Here's how the part is built. I have some questions about the finished solid (model axes, mm). Face numbers are marked on the shaded views. Coordinates: 2 decimals unless noted, no trailing zeros. Write each loop counter-clockwise with the first axis right and the second up, starting at its lowest first coordinate (ties: lowest second). Pieces come first, ordered by that corner, then holes. Notation, with made-up numbers: M 15.25,-20 L 27.25,-20 A15 ccw 27.25,-2 Z; hole C 12.5,47.25 d6. An arc over 180 degrees is marked long. Use a Markdown table: item, result.
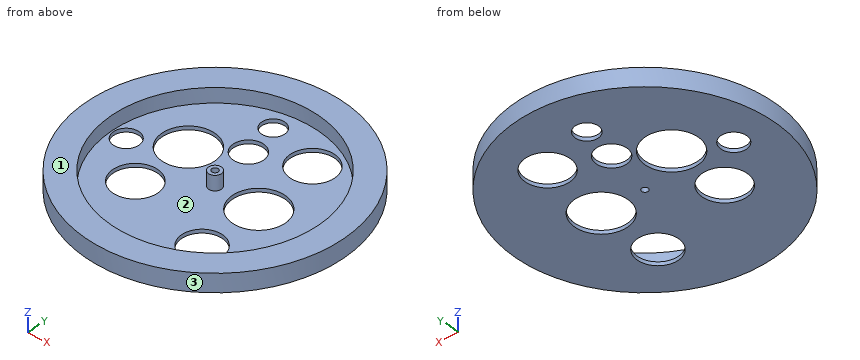
```python
from build123d import *

# Parameters (mm, degrees)
F0_R      = 70.662875
F1_DEPTH  = 10
F2_R      = 56.784897
F3_DEPTH  = 8
F4_R      = 14.477715
F5_DEPTH  = 8
F6_R      = 12.226907
F7_DEPTH  = 8
F8_R      = 7.014045
F9_DEPTH  = 8
F10_R     = 14.443937
F11_DEPTH = 8
F13_R     = 6.303091
F14_DEPTH = 8
F15_R     = 8.317638
F16_DEPTH = 8
F17_R     = 6.025281
F18_DEPTH = 8
F19_R     = 11.209177
F20_DEPTH = 8
F12_R     = 3.5
F21_DEPTH = 8
F23_D     = 3.5
F24_R     = 12.274082
F25_DEPTH = 8


with BuildPart() as f1:
    # F0 (on Top) → F1 (new body)
    with BuildSketch(Plane.XY):
        Circle(F0_R)
    extrude(amount=F1_DEPTH)

    # F2 (on face) → F3 (cut)
    with BuildSketch(Plane.XY.offset(10)):
        Circle(F2_R)
    extrude(amount=-F3_DEPTH, mode=Mode.SUBTRACT)

    # F4 (on face) → F5 (cut)
    with BuildSketch(Plane.XY.offset(2)):
        with Locations((-25.900649, 12.583426)):
            Circle(F4_R)
    extrude(amount=-F5_DEPTH, mode=Mode.SUBTRACT)

    # F6 (on face) → F7 (cut)
    with BuildSketch(Plane.XY.offset(2)):
        with Locations((20.854684, 36.710624)):
            Circle(F6_R)
    extrude(amount=-F7_DEPTH, mode=Mode.SUBTRACT)

    # F8 (on face) → F9 (cut)
    with BuildSketch(Plane.XY.offset(2)):
        with Locations((-48.892226, 0)):
            Circle(F8_R)
    extrude(amount=-F9_DEPTH, mode=Mode.SUBTRACT)

    # F10 (on face) → F11 (cut)
    with BuildSketch(Plane.XY.offset(2)):
        with Locations((24.09202, 0)):
            Circle(F10_R)
    extrude(amount=-F11_DEPTH, mode=Mode.SUBTRACT)

    # F13 (on face) → F14 (cut)
    with BuildSketch(Plane.XY.offset(2)):
        with Locations((-8.595636, 45.51062)):
            Circle(F13_R)
    extrude(amount=-F14_DEPTH, mode=Mode.SUBTRACT)

    # F15 (on face) → F16 (cut)
    with BuildSketch(Plane.XY.offset(2)):
        with Locations((-5.225664, 26.43148)):
            Circle(F15_R)
    extrude(amount=-F16_DEPTH, mode=Mode.SUBTRACT)

    # F17 (on Top) → F18 (cut)
    with BuildSketch(Plane.XY):
        with Locations((14.564808, -20.261167)):
            Circle(F17_R)
    extrude(amount=-F18_DEPTH, mode=Mode.SUBTRACT)

    # F19 (on face) → F20 (cut)
    with BuildSketch(Plane.XY.offset(2)):
        with Locations((23.249339, -34.03841)):
            Circle(F19_R)
    extrude(amount=-F20_DEPTH, mode=Mode.SUBTRACT)

    # F12 (on face) → F21 (join)
    with BuildSketch(Plane.XY.offset(2)):
        Circle(F12_R)
    extrude(amount=F21_DEPTH)

    # F23 (through all)
    with Locations(Plane.XY.offset(10)):
        with Locations((0, 0)):
            Hole(F23_D / 2)

    # F24 (on face) → F25 (cut)
    with BuildSketch(Plane.XY.offset(2)):
        with Locations((-26.544379, -19.407054)):
            Circle(F24_R)
    extrude(amount=-F25_DEPTH, mode=Mode.SUBTRACT)


solid = f1.part
```
1. Suppose I cut it at A-A on x = 0. Write out the boundary of the cut face in (y, z).
Answers follow:
| item | result |
|---|---|
| outline | M -70.66,0 L -1.75,0 L -1.75,10 L -3.5,10 L -3.5,2 L -56.78,2 L -56.78,10 L -70.66,10 Z; M 1.75,0 L 19.96,0 L 19.96,2 L 3.5,2 L 3.5,10 L 1.75,10 Z; M 32.9,0 L 70.66,0 L 70.66,10 L 56.78,10 L 56.78,2 L 32.9,2 Z |
2. I need wall thicknesses on probe 1 along X at (y, z) = (32, 0.75); probe 2 along Z at (x, y) = (-28, -33.5); probe 3 along X at (y, z) = (-32, 7.25). Which ranges of each line are inside material? Lowest first, please.
Answers follow:
| item | result |
|---|---|
| probe 1 | x = -63 to -11.4, 0.95 to 9.57, 32.14 to 63 |
| probe 2 | z = 0 to 2 |
| probe 3 | x = -63 to -46.91, 46.91 to 63 |
3. Suppose I cut it at B-B on y = 0. Write out the boundary of the cut face in (x, z), and give its area (3 significant figures).
Answers follow:
| item | result |
|---|---|
| outline | M -70.66,0 L -55.91,0 L -55.91,2 L -56.78,2 L -56.78,10 L -70.66,10 Z; M -41.88,0 L -33.06,0 L -33.06,2 L -41.88,2 Z; M -18.74,0 L -1.75,0 L -1.75,10 L -3.5,10 L -3.5,2 L -18.74,2 Z; M 1.75,0 L 9.65,0 L 9.65,2 L 3.5,2 L 3.5,10 L 1.75,10 Z; M 38.54,0 L 70.66,0 L 70.66,10 L 56.78,10 L 56.78,2 L 38.54,2 Z |
| area | 411 mm2 |
4. Suppose I cut it at C-C on y = 33. Write out the boundary of the cut face in (x, z).
Answers follow:
| item | result |
|---|---|
| outline | M -62.48,0 L -10.33,0 L -10.33,2 L -46.21,2 L -46.21,10 L -62.48,10 Z; M -0.12,0 L 9.2,0 L 9.2,2 L -0.12,2 Z; M 32.5,0 L 62.48,0 L 62.48,10 L 46.21,10 L 46.21,2 L 32.5,2 Z |
5. Suppose I cut it at D-D on x = -34.5. Write out the boundary of the cut face in (y, z), and give its area (3 significant figures).
Answers follow:
| item | result |
|---|---|
| outline | M -61.67,0 L -28.75,0 L -28.75,2 L -45.1,2 L -45.1,10 L -61.67,10 Z; M -10.06,0 L 0.94,0 L 0.94,2 L -10.06,2 Z; M 24.23,0 L 61.67,0 L 61.67,10 L 45.1,10 L 45.1,2 L 24.23,2 Z |
| area | 428 mm2 |
6. Will these pins go through, and if not, where does the flat tip stop? pin 1 Ø10 at (x, y) = (-16, -13) entering from +Z; pin 2 Ø1 at (y, z) = (-51.5, 7) entering from +X; pin 3 Ø6 at (x, z) = (50.5, 7) entering from +Y.
Answers follow:
| item | result |
|---|---|
| pin 1 | stops at z = 2 |
| pin 2 | stops at x = 48.91 |
| pin 3 | stops at y = 52.32 |
7. We'd pull the mould along Y, two halves only. Please class the marked faces 1, 2 and 3: +Y half, -Y half, draft (parallel to the pull), parting line (faces both ways), or undercut.
Answers follow:
| item | result |
|---|---|
| face 1 | draft |
| face 2 | undercut |
| face 3 | parting line |
